Can you work these out from the model? Positions are in its coordinate system, mm. Round coordinates to 2 decimals unless told otherwise and drop trailing zeros. Order: outer loops, then holes, each group sorted by start corner. A loop starts at its lowest first (then second) coordinate and runs counter-clockwise, first axis right, second up.
Q1. We'd pull the mould along Y, two halves only. Please class faces 1 (the face through (-5.618, 69.455, 0.74)), 2 (the face through (-8.746, 71.37, 0.76)), 3 (the face through (31, 22, 0)): pulls with the +Y half, pulls with the -Y half, needs draft (parallel to the pull), parting line crosses it, or undercut.
Q2. If we section it at A-A (y = 56): Please give me the cut outline in (x, z).
Q3. If I drill on line 1 (X direction, y = 14, z = 0.55); line 2 (Y direction, x = -5, z = 1.05); line 3 (Y direction, x = 5.5, z = 1.25), over which ranges is the centre line in solid material (lowest first)?
Q4. Will these pins go through, and if not, where does the flat tip stop? P1, Ø0.8, axis at x = 30.5, z = 0.5, coming from the +Y side; P2, Ø4.5, axis at x = -5.25, y = 67.8, coming from the -Z side; P3, Ø5, axis at x = 50, y = 8.5, coming from the +Z side.
Q5. If we section it at D-D (x = 14): Please give me the cut outline in (y, z).
Q6. If we section it at C-C (y = 10): Please give me the cut outline in (x, z), plus the area to 4 significant figures.
Q7. If we section it at B-B (x = 27): Please give me the cut outline in (y, z).
Autodesk Fusion 360 part; units mm, degrees
sketch "plate-2025-12-30T20_28_05.150Z" plane through (0, 0, 0) normal (0, 0, 1) x (1, 0, 0)
  line L0 (5.2708, 37.2959) -> (18.2708, 37.2959)
  line L1 (5.2708, 23.2959) -> (18.2708, 23.2959)
  line L2 (4.7708, 36.7959) -> (4.7708, 23.7959)
  line L3 (18.7708, 36.7959) -> (18.7708, 23.7959)
  arc A0 (5.2708, 37.2959) -> (4.7708, 36.7959) centre (5.2708, 36.7959) ccw
  arc A1 (18.7708, 36.7959) -> (18.2708, 37.2959) centre (18.2708, 36.7959) ccw
  arc A2 (4.7708, 23.7959) -> (5.2708, 23.2959) centre (5.2708, 23.7959) ccw
  arc A3 (18.2708, 23.2959) -> (18.7708, 23.7959) centre (18.2708, 23.7959) ccw
  line L4 (24.3208, 37.2959) -> (37.3208, 37.2959)
  line L5 (24.3208, 23.2959) -> (37.3208, 23.2959)
  line L6 (23.8208, 36.7959) -> (23.8208, 23.7959)
  line L7 (37.8208, 36.7959) -> (37.8208, 23.7959)
  arc A4 (24.3208, 37.2959) -> (23.8208, 36.7959) centre (24.3208, 36.7959) ccw
  arc A5 (37.8208, 36.7959) -> (37.3208, 37.2959) centre (37.3208, 36.7959) ccw
  arc A6 (23.8208, 23.7959) -> (24.3208, 23.2959) centre (24.3208, 23.7959) ccw
  arc A7 (37.3208, 23.2959) -> (37.8208, 23.7959) centre (37.3208, 23.7959) ccw
  line L8 (43.3708, 37.2959) -> (56.3708, 37.2959)
  line L9 (43.3708, 23.2959) -> (56.3708, 23.2959)
  line L10 (42.8708, 36.7959) -> (42.8708, 23.7959)
  line L11 (56.8708, 36.7959) -> (56.8708, 23.7959)
  arc A8 (43.3708, 37.2959) -> (42.8708, 36.7959) centre (43.3708, 36.7959) ccw
  arc A9 (56.8708, 36.7959) -> (56.3708, 37.2959) centre (56.3708, 36.7959) ccw
  arc A10 (42.8708, 23.7959) -> (43.3708, 23.2959) centre (43.3708, 23.7959) ccw
  arc A11 (56.3708, 23.2959) -> (56.8708, 23.7959) centre (56.3708, 23.7959) ccw
  line L12 (5.2708, 18.2459) -> (18.2708, 18.2459)
  line L13 (5.2708, 4.2459) -> (18.2708, 4.2459)
  line L14 (4.7708, 17.7459) -> (4.7708, 4.7459)
  line L15 (18.7708, 17.7459) -> (18.7708, 4.7459)
  arc A12 (5.2708, 18.2459) -> (4.7708, 17.7459) centre (5.2708, 17.7459) ccw
  arc A13 (18.7708, 17.7459) -> (18.2708, 18.2459) centre (18.2708, 17.7459) ccw
  arc A14 (4.7708, 4.7459) -> (5.2708, 4.2459) centre (5.2708, 4.7459) ccw
  arc A15 (18.2708, 4.2459) -> (18.7708, 4.7459) centre (18.2708, 4.7459) ccw
  line L16 (24.3208, 18.2459) -> (37.3208, 18.2459)
  line L17 (24.3208, 4.2459) -> (37.3208, 4.2459)
  line L18 (23.8208, 17.7459) -> (23.8208, 4.7459)
  line L19 (37.8208, 17.7459) -> (37.8208, 4.7459)
  arc A16 (24.3208, 18.2459) -> (23.8208, 17.7459) centre (24.3208, 17.7459) ccw
  arc A17 (37.8208, 17.7459) -> (37.3208, 18.2459) centre (37.3208, 17.7459) ccw
  arc A18 (23.8208, 4.7459) -> (24.3208, 4.2459) centre (24.3208, 4.7459) ccw
  arc A19 (37.3208, 4.2459) -> (37.8208, 4.7459) centre (37.3208, 4.7459) ccw
  line L20 (43.3708, 18.2459) -> (56.3708, 18.2459)
  line L21 (43.3708, 4.2459) -> (56.3708, 4.2459)
  line L22 (42.8708, 17.7459) -> (42.8708, 4.7459)
  line L23 (56.8708, 17.7459) -> (56.8708, 4.7459)
  arc A20 (43.3708, 18.2459) -> (42.8708, 17.7459) centre (43.3708, 17.7459) ccw
  arc A21 (56.8708, 17.7459) -> (56.3708, 18.2459) centre (56.3708, 17.7459) ccw
  arc A22 (42.8708, 4.7459) -> (43.3708, 4.2459) centre (43.3708, 4.7459) ccw
  arc A23 (56.3708, 4.2459) -> (56.8708, 4.7459) centre (56.3708, 4.7459) ccw
  line L24 (-10.2492, 72.7959) -> (72.6508, 72.7959)
  line L25 (72.6508, 72.7959) -> (72.6508, -10.6041)
  line L26 (72.6508, -10.6041) -> (-10.2492, -10.6041)
  line L27 (-10.2492, -10.6041) -> (-10.2492, 72.7959)
  line L28 (22.6008, 72.7959) -> (41.1008, 72.7959)
  line L29 (41.1008, 72.7959) -> (41.1008, 41.7959)
  line L30 (41.1008, 41.7959) -> (22.6008, 41.7959)
  line L31 (22.6008, 41.7959) -> (22.6008, 72.7959)
  circle A24 centre (-5.2492, 67.7959) radius 1.7
  circle A25 centre (-5.2492, -5.6041) radius 1.7
  circle A26 centre (67.6508, -5.6041) radius 1.7
  circle A27 centre (67.6508, 67.7959) radius 1.7
  dimension "d1" = 82.9
  dimension "d2" = 83.4
  dimension "d3" = 15.02
  dimension "d4" = 14.85
  dimension "d5" = 18.5
  dimension "d6" = 31
  dimension "d7" = 32.85
  dimension "d8" = 3.4
  dimension "d9" = 5
  dimension "d10" = 5
  dimension "d11" = 3.4
  dimension "d12" = 5
  dimension "d13" = 5
  dimension "d14" = 3.4
  dimension "d15" = 5
  dimension "d16" = 5
  dimension "d17" = 3.4
  dimension "d18" = 5
  dimension "d19" = 5
extrude "Extrude1" add sketch "plate-2025-12-30T20_28_05.150Z" along normal blind 1.5 contours L24 L25 L26 L27 L29 L30 L31
fillet "Fillet1" radius 5 4 edges at (72.6508, -10.6041, 0.75) (72.6508, 72.7959, 0.75) (-10.2492, 72.7959, 0.75) (-10.2492, -10.6041, 0.75)
Solution:
1. face 1: undercut
1. face 2: pulls with the +Y half
1. face 3: needs draft
2. outline: (-10.25, 0) - (22.6, 0) - (22.6, 1.5) - (-10.25, 1.5) - close; (41.1, 0) - (72.65, 0) - (72.65, 1.5) - (41.1, 1.5) - close
3. line 1: x = -10.25 to 4.77, 18.77 to 23.82, 37.82 to 42.87, 56.87 to 72.65
3. line 2: y = -10.6 to -7.29, -3.92 to 66.11, 69.48 to 72.8
3. line 3: y = -10.6 to 4.25, 18.25 to 23.3, 37.3 to 72.8
4. P1: stops at y = 41.8
4. P2: stops at z = 0
4. P3: passes through
5. outline: (-10.6, 0) - (4.25, 0) - (4.25, 1.5) - (-10.6, 1.5) - close; (18.25, 0) - (23.3, 0) - (23.3, 1.5) - (18.25, 1.5) - close; (37.3, 0) - (72.8, 0) - (72.8, 1.5) - (37.3, 1.5) - close
6. outline: (-10.25, 0) - (4.77, 0) - (4.77, 1.5) - (-10.25, 1.5) - close; (18.77, 0) - (23.82, 0) - (23.82, 1.5) - (18.77, 1.5) - close; (37.82, 0) - (42.87, 0) - (42.87, 1.5) - (37.82, 1.5) - close; (56.87, 0) - (72.65, 0) - (72.65, 1.5) - (56.87, 1.5) - close
6. area: 61.35 mm2
7. outline: (-10.6, 0) - (4.25, 0) - (4.25, 1.5) - (-10.6, 1.5) - close; (18.25, 0) - (23.3, 0) - (23.3, 1.5) - (18.25, 1.5) - close; (37.3, 0) - (41.8, 0) - (41.8, 1.5) - (37.3, 1.5) - close
